from build123d import *

# Parameters (mm, degrees)
PAD001_DEPTH    = 23
SKETCH003_R     = 2.25
POCKET_DEPTH    = 5
SKETCH004_R     = 2.25
POCKET001_DEPTH = 5


with BuildPart() as part:
    # Sketch001 → Pad001 (new body)
    with BuildSketch(Plane.XZ):
        with BuildLine():
            Line((56.25, -75), (56.25, 75))
            Line((56.25, 75), (-56.25, 75))
            Line((-56.25, 75), (-41.25, 55))
            ThreePointArc((41.25, -55), (22.420595, 16.815446), (-41.25, 55))
            Line((41.25, -55), (56.25, -75))
        make_face()
    extrude(amount=PAD001_DEPTH)

    # Sketch003 (on Face2 of Pad001) → Pocket (cut)
    with BuildSketch(Plane(origin=(56.25, 0, 0), x_dir=(0, 0, 1), z_dir=(1, 0, 0))):
        with Locations((-45, 11.5)):
            Circle(SKETCH003_R)
        with Locations((45, 11.5)):
            Circle(SKETCH003_R)
    extrude(amount=-POCKET_DEPTH, mode=Mode.SUBTRACT)

    # Sketch004 (on Face7 of Pocket) → Pocket001 (cut)
    with BuildSketch(Plane(origin=(0, 0, 75), x_dir=(-1, 0, 0), z_dir=(0, 0, 1))):
        with Locations((-33.75, 11.5)):
            Circle(SKETCH004_R)
        with Locations((33.75, 11.5)):
            Circle(SKETCH004_R)
    extrude(amount=-POCKET001_DEPTH, mode=Mode.SUBTRACT)


solid = part.part
Work out the finished part from the listing and answer in its coordinate system (mm). A direction names the side the tool comes from. Round coordinates to 2 decimals unless told otherwise and drop trailing zeros. Order: outer loops, then holes, each group sorted by start corner. A loop starts at its lowest first (then second) coordinate and runs counter-clockwise, first axis right, second up. Notation, with made-up numbers: M -11,50 L 26,50 A15 cw 26,55 Z; hole C -23,-28 d9. An arc over 180 degrees is marked long. Put each result on its own line as item: value. Start each with the question number.
Q1. Section B-B, the plane x = -33.75 is taken. Write down the section's boundary in (y, z), and give its area (3 significant figures).
Q2. Flat-ended cylindrical pins translate along their axes: pin 1 (6 mm diameter, centred on x = -33.75, y = -11.5, fed in from -Z); pin 2 (2 mm diameter, centred on x = -33.5, y = -11, fed in from +Z); pin 3 (2.5 mm diameter, centred on y = -11.5, z = -45, fed in from -X). Find the tip coordinate at first contact, or state that the pin passes through.
Q3. Section A-A, the plane y = -11.5 is taken. Write down the section's boundary in (x, z), and give its area (4 significant figures).
Q4. A tool of negligible diameter and unlimited length cuts with its end or side. For faces 1 (the flat face through (-48.855, -11.339, 65.14)), 2 (the flat face through (34, -12, 70)), 3 (the cylindrical face through (53.785, -11.599, -47.248)), from which of +Z, -Z, +X, -X, +Y, -Y can it reach the whole face along a straight path? Write none if from no direction.
Q5. Section D-D, the plane x = 11 is taken. Write down the section's boundary in (y, z), and give its area (3 significant figures).
Q6. For a pull along Y with two mould halves and no side action, classify faces 4 (the flat face through (25, -23, 34)), 5 (the flat face through (48.645, -11.339, -64.86)), 6 (the cylindrical face through (53.785, -11.599, 42.752)) as pulls with the +Y half, pulls with the -Y half, needs draft (parallel to the pull), parting line crosses it, or undercut.
Q7. Section C-C, the plane z = 45 is taken. Write down the section's boundary in (x, y), and give its area (3 significant figures).
Q8. Straight lines are drawn through the part: L1, parallel to Y at x = 55, z = -45; L2, parallel to X at y = -11.5, z = 71.9 (3 decimals); L3, parallel to Y at x = -33, z = 73. For each, find the intervals that lie inside material, in ascending order. Write a range as [from, to].
Findings below:
1. outline: M -23,53.54 L 0,53.54 L 0,75 L -9.25,75 L -9.25,70 L -13.75,70 L -13.75,75 L -23,75 Z
1. area: 471 mm^2
2. pin 1: stops at z = 52.79
2. pin 2: stops at z = 70
2. pin 3: stops at x = 42
3. outline: M -56.25,75 L -41.25,55 A98.34 cw 41.25,-55 L 56.25,-75 L 56.25,-47.25 L 51.25,-47.25 L 51.25,-42.75 L 56.25,-42.75 L 56.25,42.75 L 51.25,42.75 L 51.25,47.25 L 56.25,47.25 L 56.25,75 L 36,75 L 36,70 L 31.5,70 L 31.5,75 L -31.5,75 L -31.5,70 L -36,70 L -36,75 Z
3. area: 5,695 mm^2
4. face 1: -Z, -X, +Y, -Y
4. face 2: +Z
4. face 3: +X
5. outline: M -23,29.56 L 0,29.56 L 0,75 L -23,75 Z
5. area: 1,050 mm^2
6. face 4: pulls with the -Y half
6. face 5: needs draft
6. face 6: undercut
7. outline: M -10.77,-23 L 56.25,-23 L 56.25,-13.75 L 51.25,-13.75 L 51.25,-9.25 L 56.25,-9.25 L 56.25,0 L -10.77,0 Z
7. area: 1,520 mm^2
8. L1: y = [-23, -13.75], [-9.25, 0]
8. L2: x = [-53.925, -36], [-31.5, 31.5], [36, 56.25]
8. L3: y = [-23, -13.62], [-9.38, 0]
